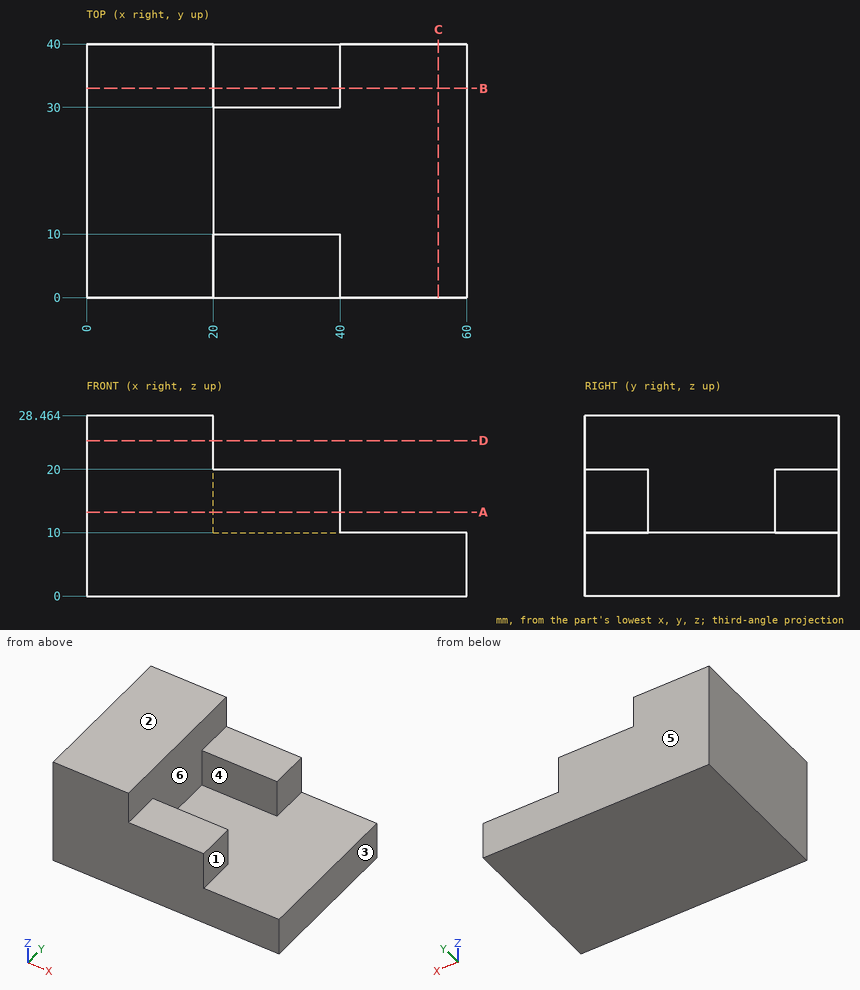
Study the drawing (mm; zero at the part's minimum x, y, z) and answer. A direction names the side the tool comes from. Round coordinates to 2 decimals unless told otherwise and drop trailing zeros. Loops run counter-clockwise (first coordinate to the right, second up) from the corner with the lowest first, then second, coordinate; pieces in that order, holes last.
Q1. Section B-B, the plane y = 33 is taken. Determine the outline of the cut face in (x, z).
Q2. Section A-A, the plane z = 13.25 is taken. Determine the outline of the cut face in (x, y).
Q3. Given pin 1 Ø6 at (x, y) = (38, 23.5) entering from -Z; pin 2 Ø11 at (x, y) = (26.5, 34) entering from +Z; pin 3 Ø9 at (y, z) = (20.5, 19) entering from +X; pin 4 Ø8 at (x, y) = (30, 25.5) entering from +Z, each flat-ended and moving along its own axis, determine where each tip first touches the part or whether it passes through.
Q4. Find the intervals of material crossed by line 1 (Z direction, x = 43.5, y = 28); line 2 (Y direction, x = 36, z = 19); line 3 (X direction, y = 33.5, z = 17.25), in increasing order.
Q5. Section C-C, the plane x = 55.5 is taken. Determine the outline of the cut face in (y, z).
Q6. For a pull along Y with two mould halves and no side action, classify the marked faces 3, 4, 5 and 6 as released by +Y, released by -Y, zero draft, split by the parting line, or undercut.
Q7. Which of the six approach directions +Z, -Z, +X, -X, +Y, -Y give full straight-line access (tool end or side, diameter ignored) to the marked faces 1 and 2?
Q8. Section D-D, the plane z = 24.5 is taken. Determine the outline of the cut face in (x, y).
Completed:
1. outline: (0, 0) - (60, 0) - (60, 10) - (40, 10) - (40, 20) - (20, 20) - (20, 28.46) - (0, 28.46) - close
2. outline: (0, 0) - (40, 0) - (40, 10) - (20, 10) - (20, 30) - (40, 30) - (40, 40) - (0, 40) - close
3. pin 1: stops at z = 0
3. pin 2: stops at z = 20
3. pin 3: stops at x = 20
3. pin 4: stops at z = 10
4. line 1: z = 0 to 10
4. line 2: y = 0 to 10, 30 to 40
4. line 3: x = 0 to 40
5. outline: (0, 0) - (40, 0) - (40, 10) - (0, 10) - close
6. face 3: zero draft
6. face 4: undercut
6. face 5: released by +Y
6. face 6: undercut
7. face 1: +Z, +X, +Y, -Y
7. face 2: +Z, +X, -X, +Y, -Y
8. outline: (0, 0) - (20, 0) - (20, 40) - (0, 40) - close
